```python
from build123d import *

# Parameters (mm, degrees)
SKETCH1_R           = 1.5
BOSS_EXTRUDE1_DEPTH = 3.18


with BuildPart() as part:
    # Sketch1 → Boss-Extrude1 (new body)
    with BuildSketch(Plane.XY):
        Polygon((-103.18, 100), (-12.5, 100), (-12.5, 103.18), (12.5, 103.18), (12.5, 100), (103.18, 100), (103.18, 12.5), (100, 12.5), (100, 1.5), (96, 1.5), (96, 3), (93, 3), (93, 1.5), (90.18, 1.5), (90.18, -1.5), (93, -1.5), (93, -3), (96, -3), (96, -1.5), (100, -1.5), (100, -12.5), (103.18, -12.5), (103.18, -100), (12.5, -100), (12.5, -103.18), (-12.5, -103.18), (-12.5, -100), (-103.18, -100), (-103.18, -12.5), (-100, -12.5), (-100, -1.5), (-96, -1.5), (-96, -3), (-93, -3), (-93, -1.5), (-90.18, -1.5), (-90.18, 1.5), (-93, 1.5), (-93, 3), (-96, 3), (-96, 1.5), (-100, 1.5), (-100, 12.5), (-103.18, 12.5), align=None)
        with Locations(Location((0, -101.59, 0), (0, 0, 180))):
            Circle(SKETCH1_R, mode=Mode.SUBTRACT)
        with Locations(Location((0, 101.59, 0), (0, 0, 180))):
            Circle(SKETCH1_R, mode=Mode.SUBTRACT)
    extrude(amount=BOSS_EXTRUDE1_DEPTH)


solid = part.part
```
Build history of the part. All positions in model axes, mm. Give positions to 0.01 mm unless a question says otherwise; leave off trailing zeros. Loops run counter-clockwise (first coordinate to the right, second up) from the corner with the lowest first, then second, coordinate; pieces in that order, holes last.
1) Band-saw the part on B-B on z = 1.5. State how many separate pieces and enclosed holes the cut face has, then the cut area to 3 significant figures.
Values follow:
separate pieces: 1
enclosed holes: 2
area: 41,200 mm2
2) Drop flat-ended pins along their axis: P1, Ø5, axis at x = 25.5, y = -58, coming from the -Z side; P2, Ø1, axis at x = 51, z = 2, coming from the +Y side; P3, Ø1.5, axis at x = 94, z = 1.5, coming from the -Y side; P4, Ø1.8, axis at x = 0, y = 101.59, coming from the +Z side. Give the stop position or say it passes through.
Values follow:
P1: stops at z = 0
P2: stops at y = 100
P3: stops at y = -100
P4: passes through
3) Band-saw the part on A-A on x = -73. List the corners of the cut face in (y, z).
Values follow:
outline: (-100, 0) - (100, 0) - (100, 3.18) - (-100, 3.18) - close
4) Probe line 1 along X through (y, z) = (101.59, 1.05); line 2 along Y through (x, z) = (-94, 2.4); line 3 along Y through (x, z) = (14, 0.45). List the from-to ranges inside material, lowest first.
Values follow:
line 1: x = -12.5 to -1.5, 1.5 to 12.5
line 2: y = -100 to -3, 3 to 100
line 3: y = -100 to 100
